Build history of the part. All positions in model axes, mm. Give positions to 0.01 mm unless a question says otherwise; leave off trailing zeros. Write each loop counter-clockwise with the first axis right and the second up, starting at its lowest first coordinate (ties: lowest second). Pieces come first, ordered by that corner, then holes. Notation, with made-up numbers: (82, 41) - (104, 41) arc R18 cw to (104, 53) - close; hole circle Ø10 at (66.25, 54.5). An arc over 180 degrees is marked (long way). Use one line per item in the form item = value. Start each with the question number.
Autodesk Inventor part; units mm, degrees
ref_plane "YZ Plane" through (0, 0, 0) normal (1, 0, 0) x (0, 1, 0)
ref_plane "XZ Plane" through (0, 0, 0) normal (0, 1, 0) x (-1, 0, 0)
ref_plane "XY Plane" through (0, 0, 0) normal (0, 0, 1) x (1, 0, 0)
sketch "Sketch1" plane through (0, 0, 0) normal (0, 0, 1) x (1, 0, 0)
  line L0 (0, 0) -> (38.1, 0)
  line L1 (38.1, 0) -> (38.1, -85.725)
  line L2 (38.1, -85.725) -> (0, -85.725)
  line L3 (0, -85.725) -> (0, 0)
  line L4 (38.1, -85.725) -> (38.1, -123.825)
  line L5 (38.1, -123.825) -> (0, -85.725)
  dimension "d0" = 38.1
  dimension "d1" = 85.725
  dimension "d4" = 38.1
extrude "Extrusion1" add sketch "Sketch1" along normal blind 0.4039 contours L0 L1 L2 L3
extrude "Extrusion2" add sketch "Sketch1" along normal blind 0.4039 contours L2 L4 L5
sketch "Sketch2" plane through (0, 0, 0.4039) normal (0, 0, 1) x (1, 0, 0)
  line L0 (0, -85.725) -> (38.1, -123.825)
  line L1 (38.1, -123.825) -> (38.1, 0)
  line L2 (38.1, -113.0487) -> (5.3882, -80.3368)
  line L3 (0, -85.725) -> (5.3882, -80.3368)
  line L4 (38.1, -113.0487) -> (38.1, -123.825)
  line L5 (38.1, -123.825) -> (0, -85.725)
  line L6 (0, -85.725) -> (5.3882, -80.3368)
  line L7 (5.3882, -80.3368) -> (38.1, -113.0487)
  line L8 (38.1, -113.0487) -> (38.1, -123.825)
  line L9 (38.1, -123.825) -> (0, -85.725)
  dimension "d7" = 7.62
extrude "Extrusion3" cut sketch "Sketch2" against normal blind 25.4
sketch "Sketch3" plane through (0, 0, 0) normal (0, 0, -1) x (-1, 0, 0)
  circle A0 centre (-25.4, -15.24) radius 1.4986
  circle A1 centre (-25.4, -76.2) radius 1.4986
  line L0 (0, 0) -> (-38.1, 0)
  line L1 (-38.1, 0) -> (-38.1, -113.0487)
  dimension "d19" = 2.9972
  dimension "d20" = 15.24
  dimension "d21" = 12.7
  dimension "d22" = 12.7
extrude "Extrusion4" cut sketch "Sketch3" against normal blind 25.4
properties part number "Plate_InnerSide_Alu25" material "Aluminum 6061"
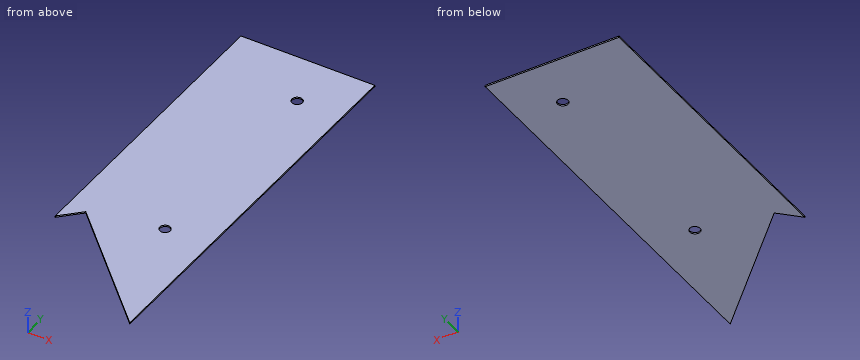
(1) Cut at C-C, the plane x = 25.4. Give the cut face in (y, z).
(2) Wall check: line 1 (X direction, y = -76.2, z = 0.1); line 2 (Y direction, x = 25.4, z = 0.2); line 3 (Y direction, x = 34, z = 0.3). Give the ranges that are in metal, low to high. Write a range as from..to.
(3) Cut at B-B, the plane y = -15.24. Give the cut face in (x, z), then the cut area to 3 significant figures.
(4) Cut at D-D, the plane x = 31.5. Give the cut face in (y, z), then the cut area to 3 significant figures.
(5) Cut at A-A, the plane z = 0.3. Give the cut face in (x, y) (3 decimals).
Solution:
q1.outline = (-100.35, 0) - (-77.7, 0) - (-77.7, 0.4) - (-100.35, 0.4) - close; (-74.7, 0) - (-16.74, 0) - (-16.74, 0.4) - (-74.7, 0.4) - close; (-13.74, 0) - (0, 0) - (0, 0.4) - (-13.74, 0.4) - close
q2.line_1 = 0..23.9, 26.9..38.1
q2.line_2 = -100.35..-77.7, -74.7..-16.74, -13.74..0
q2.line_3 = -108.95..0
q3.outline = (0, 0) - (23.9, 0) - (23.9, 0.4) - (0, 0.4) - close; (26.9, 0) - (38.1, 0) - (38.1, 0.4) - (26.9, 0.4) - close
q3.area = 14.2 mm2
q4.outline = (-106.45, 0) - (0, 0) - (0, 0.4) - (-106.45, 0.4) - close
q4.area = 43.0 mm2
q5.outline = (0, -85.725) - (5.388, -80.337) - (38.1, -113.049) - (38.1, 0) - (0, 0) - close; hole circle Ø2.997 at (25.4, -76.2); hole circle Ø2.997 at (25.4, -15.24)
